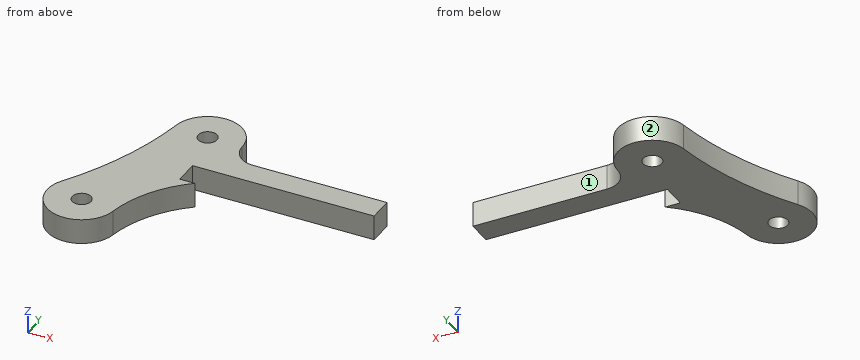
```python
from build123d import *

# Parameters (mm, degrees)
SKETCH1_R           = 1.5
BOSS_EXTRUDE1_DEPTH = 4
SKETCH2_W           = 29
SKETCH2_H           = 4
CUT_EXTRUDE1_DEPTH  = 10


with BuildPart() as part:
    # Sketch1 → Boss-Extrude1 (new body)
    with BuildSketch(Plane.XY):
        with BuildLine():
            Line((30.5, -3.6), (9.1, -3.6))
            ThreePointArc((9.1, -3.6), (6.554415588, -2.545584412), (5.5, 0))
            ThreePointArc((5.5, 0), (0.421431882, 5.483830337), (-5.435416425, 0.840385797))
            ThreePointArc((-5.435416425, 0.840385797), (-8.227950432, -9.8038682), (-13.142048472, -19.650188822))
            ThreePointArc((-13.142048472, -19.650188822), (-10.445387128, -27.744460023), (-3.067628607, -23.459849435))
            ThreePointArc((-3.067628607, -23.459849435), (3.290458074, -12.104682623), (15.5, -7.6))
            Line((15.5, -7.6), (30.5, -7.6))
            Line((30.5, -7.6), (30.5, -3.6))
        make_face()
        Circle(SKETCH1_R, mode=Mode.SUBTRACT)
        with Locations((-8.5, -22.6)):
            Circle(SKETCH1_R, mode=Mode.SUBTRACT)
    extrude(amount=BOSS_EXTRUDE1_DEPTH)

    # Sketch2 → Cut-Extrude1 (cut)
    with BuildSketch(Plane.XY.offset(4)):
        with Locations((16, -9.6)):
            Rectangle(SKETCH2_W, SKETCH2_H)
    extrude(amount=-CUT_EXTRUDE1_DEPTH, mode=Mode.SUBTRACT)


solid = part.part
```
Geometry: final body of the model. Coordinates: model frame, mm. Face numbers are marked on the shaded views. A direction names the side the tool comes from. Round coordinates to 2 decimals unless told otherwise and drop trailing zeros. Order: outer loops, then holes, each group sorted by start corner. A loop starts at its lowest first (then second) coordinate and runs counter-clockwise, first axis right, second up. Notation, with made-up numbers: (50.25, 33.5) - (104.25, 33.5) arc R16 ccw to (104.25, 59.5) - close; hole circle Ø2 at (-21, 26). An arc over 180 degrees is marked (long way). Write item = value, one per line. Start each with the question number.
Q1. Access query for the marked faces 1 and 2. Directions: +Z, -Z, +X, -X, +Y, -Y. A direction counts if a zero-diameter tool reaches every point of the face in a straight line with its end or side. Return the directions, or none.
Q2. Pin query (flat end, axial travel): pin 1 (1.5 mm diameter, centred on x = 7.5, z = 1.5, fed in from -Y); pin 2 (1.2 mm diameter, centred on x = 2.5, z = 1.5, fed in from +Y); pin 3 (1.5 mm diameter, centred on x = 15.5, z = 0.5, fed in from +Y). Return the tip coordinate at first contact, or that it passes through.
Q3. Ray query, line 1 (Y direction, x = -8.5, z = 1); line 2 (Y direction, x = -9.5, z = 3.55); line 3 (Y direction, x = 21, z = 2.7). Return the intervals inside material, ascending. Write a range as from..to.
Q4. Cut plane D-D on x = 25. Return the cut outline in (y, z), and give its area (3 significant figures).
Q5. Cut plane C-C on z = 2.85. Return the cut outline in (x, y).
Q6. Cut plane A-A on x = -8.5. Return the cut outline in (y, z), and give its area (3 significant figures).
Q7. Cut plane B-B on y = -22.6. Return the cut outline in (x, z).
Outcome:
q1.face_1 = +Z, -Z, +X, +Y
q1.face_2 = +Z, -Z, +Y
q2.pin_1 = -7.6
q2.pin_2 = 5.16
q2.pin_3 = -3.6
q3.line_1 = -28.1..-24.1, -21.1..-10.51
q3.line_2 = -28.01..-23.72, -21.48..-12.89
q3.line_3 = -7.6..-3.6
q4.outline = (-7.6, 0) - (-3.6, 0) - (-3.6, 4) - (-7.6, 4) - close
q4.area = 16.0 mm^2
q5.outline = (-13.14, -19.65) arc R5.5 ccw (long way) to (-3.07, -23.46) arc R18.8 cw to (3.91, -11.6) - (1.5, -11.6) - (1.5, -7.6) - (30.5, -7.6) - (30.5, -3.6) - (9.1, -3.6) arc R3.6 cw to (5.5, 0) arc R5.5 ccw to (-5.44, 0.84) arc R53.43 cw to start; hole circle Ø3 at (-8.5, -22.6); hole circle Ø3 at (0, 0)
q6.outline = (-28.1, 0) - (-24.1, 0) - (-24.1, 4) - (-28.1, 4) - close; (-21.1, 0) - (-10.51, 0) - (-10.51, 4) - (-21.1, 4) - close
q6.area = 58.4 mm^2
q7.outline = (-14, 0) - (-10, 0) - (-10, 4) - (-14, 4) - close; (-7, 0) - (-2.91, 0) - (-2.91, 4) - (-7, 4) - close
